Answer from the drawing. Dimensions are ordinates in mm from the lowest x, y and z of the part. Give positions to 0.01 mm unless a question says otherwise; leave off trailing zeros. Write each loop counter-clockwise with the first axis right and the second up, starting at its lowest first coordinate (ties: lowest second). Pieces come first, ordered by that corner, then holes. Notation, with made-up numbers: (42.25, -25) -> (68.25, -25) arc R27 cw to (68.25, 6) -> close; hole circle Ø1 at (36, 64). An arc over 180 degrees is marked (long way). Write item = value, one per line.
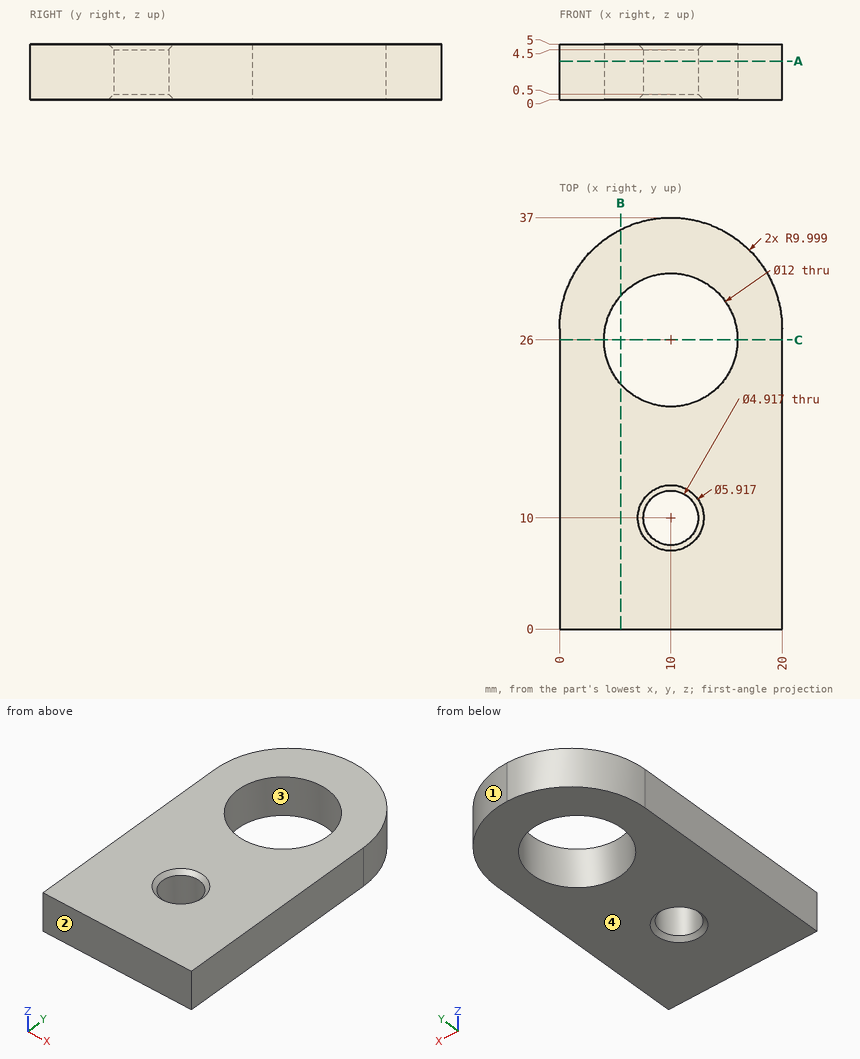
(1) The part is cut by section C-C on y = 26. Determine the outline of the cut face in (x, z), plus the area to 3 significant figures.
Checks:
outline = (0, 0) -> (4, 0) -> (4, 5) -> (0, 5) -> close; (16, 0) -> (20, 0) -> (20, 5) -> (16, 5) -> close
area = 40.0 mm²
(2) For a pull along Y with two mould halves and no side action, classify the marked faces 1, 2, 3 and 4 as released by +Y, released by -Y, zero draft, split by the parting line, or undercut.
Checks:
face_1 = released by +Y
face_2 = released by -Y
face_3 = undercut
face_4 = zero draft
(3) The part is cut by section A-A on z = 3.45. Count the separate pieces of the cut face and the enclosed holes in it, plus the area to 3 significant figures.
Checks:
separate_pieces = 1
enclosed_holes = 2
area = 565 mm²
(4) The part is cut by section B-B on x = 5.5. Determine the outline of the cut face in (y, z).
Checks:
outline = (0, 0) -> (22.03, 0) -> (22.03, 5) -> (0, 5) -> close; (29.97, 0) -> (35.93, 0) -> (35.93, 5) -> (29.97, 5) -> close
(5) Given P1, Ø2, axis at y = 5, z = 2, coming from the -X side; P2, Ø11, axis at x = 10, y = 26, coming from the -Z side; P3, Ø3, axis at y = 32, z = 3.5, coming from the +X side, each flat-ended and moving along its own axis, determine where each tip first touches the part or whether it passes through.
Checks:
P1 = 0
P2 = through
P3 = 19.37
(6) Consider L1, parallel to Y at x = 10, z = 1.45; L2, parallel to X at y = 10, z = 2.8; L3, parallel to Y at x = 5, z = 2.7 (1 decimal). Determine where each line is inside the solid, lowest interval first.
Checks:
L1 = 0 to 7.54, 12.46 to 20, 32 to 37
L2 = 0 to 7.54, 12.46 to 20
L3 = 0 to 22.7, 29.3 to 35.7
